CAD build for the part. Positions are in the model's coordinates, mm. A direction names the side the tool comes from. Round coordinates to 2 decimals unless told otherwise and drop trailing zeros. Write each loop counter-clockwise with the first axis right and the second up, starting at its lowest first coordinate (ties: lowest second). Pieces come first, ordered by that corner, then holes. Notation, with made-up numbers: (37, 48.5) -> (55, 48.5) arc R37 cw to (55, 84.5) -> close; hole circle Ø1 at (58.5, -23.5). An arc over 180 degrees is marked (long way). Put each result on its own line as item: value. Start each with the question number.
1. 3-axis set-ups, long thin cutter, end or side, ignore diameter. For faces 1 (the flat face through (49, 35, 3)), 2 (the flat face through (2.5, 18, 26)), 3 (the flat face through (6, 36, 3)), 4 (the flat face through (47, 0, 25)), 5 (the flat face through (46, 20, 48.5)): which of +Z, -Z, +X, -X, +Y, -Y reach the whole face in a straight line?
2. Saw through at B-B on z = 12.5. List the corners of the cut face in (x, y), and give its area (3 significant figures).
3. Drill centre lines: line 1 (X direction, y = 7, z = 18.5); line 2 (Z direction, x = 43, y = 17.5); line 3 (Y direction, x = 28, z = 25). Where is each one in solid material? Low to high. Write a range as from..to.
4. Saw through at A-A on y = 10.5. List the corners of the cut face in (x, z), and give its area (3 significant figures).
5. Flat gauge pins, fed straight in: P1, Ø4, axis at x = 10.5, z = 7, coming from the +Y side; P2, Ø1, axis at y = 35.5, z = 3.5, coming from the -X side; P3, Ø3, axis at x = 1.5, z = 19.5, coming from the +Y side. Where does each tip first touch, or does it go through?
6. Saw through at C-C on x = 77. List the corners of the cut face in (y, z).
7. Pull direction Y, two halves, no side cores. Call faces 6 (the flat face through (1, 33, 25)), 7 (the flat face through (49, 35, 47)), 8 (the flat face through (46, 20, 2.5)), 9 (the flat face through (6, 36, 47)): pulls with the +Y half, pulls with the -Y half, needs draft (parallel to the pull), parting line crosses it, or undercut.
from build123d import *

# Parameters (mm, degrees)
ESBO_O1_W                = 95
ESBO_O1_H                = 51
RESSALTO_EXTRUS_O1_DEPTH = 2.5
ESBO_O2_W                = 95
ESBO_O2_H                = 51
ESBO_O2_W_2              = 90
ESBO_O2_H_2              = 46
RESSALTO_EXTRUS_O3_DEPTH = 37
ESBO_O3_W                = 46
ESBO_O3_H                = 4
CORTE_EXTRUS_O3_DEPTH    = 2.5
RESSALTO_EXTRUS_O7_START = -6
ESBO_O4_W                = 2
ESBO_O4_H                = 2
RESSALTO_EXTRUS_O7_DEPTH = 86.5


with BuildPart() as part:
    # Esboço1 → Ressalto-extrusão1 (new body)
    with BuildSketch(Plane(origin=(0, 0, 0), x_dir=(1, 0, 0), z_dir=(0, 1, 0))):
        with Locations((47.5, -25.5)):
            Rectangle(ESBO_O1_W, ESBO_O1_H)
    extrude(amount=RESSALTO_EXTRUS_O1_DEPTH)

    # Esboço2 → Ressalto-extrusão3 (add)
    with BuildSketch(Plane(origin=(0, 0, 0), x_dir=(1, 0, 0), z_dir=(0, 1, 0))):
        with Locations((47.5, -25.5)):
            Rectangle(ESBO_O2_W, ESBO_O2_H)
        with Locations((47.5, -25.5)):
            Rectangle(ESBO_O2_W_2, ESBO_O2_H_2, mode=Mode.SUBTRACT)
    extrude(amount=RESSALTO_EXTRUS_O3_DEPTH)

    # Esboço3 → Corte-extrusão3 (cut)
    with BuildSketch(Plane.ZY):
        with Locations((25.5, 35)):
            Rectangle(ESBO_O3_W, ESBO_O3_H)
    extrude(amount=-CORTE_EXTRUS_O3_DEPTH, mode=Mode.SUBTRACT)

    # Esboço4 → Ressalto-extrusão7 (add)
    with BuildSketch(Plane.ZY.offset(RESSALTO_EXTRUS_O7_START)):
        with Locations((3.5, 36)):
            Rectangle(ESBO_O4_W, ESBO_O4_H)
        with Locations((47.5, 36)):
            Rectangle(ESBO_O4_W, ESBO_O4_H)
    extrude(amount=-RESSALTO_EXTRUS_O7_DEPTH)


solid = part.part
Return value:
1. face 1: -X
1. face 2: +Y
1. face 3: -X, +Y
1. face 4: +Z, -Z, +X, -X, -Y
1. face 5: none
2. outline: (0, 0) -> (95, 0) -> (95, 37) -> (92.5, 37) -> (92.5, 2.5) -> (2.5, 2.5) -> (2.5, 33) -> (0, 33) -> close
2. area: 400 mm^2
3. line 1: x = 0..2.5, 92.5..95
3. line 2: z = 0..2.5, 48.5..51
3. line 3: y = 0..2.5
4. outline: (0, 0) -> (95, 0) -> (95, 51) -> (0, 51) -> close; hole (2.5, 2.5) -> (92.5, 2.5) -> (92.5, 48.5) -> (2.5, 48.5) -> close
4. area: 705 mm^2
5. P1: stops at y = 2.5
5. P2: stops at x = 6
5. P3: stops at y = 33
6. outline: (0, 0) -> (37, 0) -> (37, 4.5) -> (35, 4.5) -> (35, 2.5) -> (2.5, 2.5) -> (2.5, 48.5) -> (35, 48.5) -> (35, 46.5) -> (37, 46.5) -> (37, 51) -> (0, 51) -> close
7. face 6: pulls with the +Y half
7. face 7: undercut
7. face 8: undercut
7. face 9: needs draft
